Check sheet for the modelled part. Datum: model origin and axes. Units: mm. Face numbers are marked on the shaded views. A direction names the side the tool comes from. Round coordinates to 2 decimals unless told otherwise and drop trailing zeros. Write each loop counter-clockwise with the first axis right and the second up, starting at its lowest first coordinate (ties: lowest second). Pieces come first, ordered by that corner, then holes. Notation, with made-up numbers: (20, 48) - (72, 48) arc R12 cw to (72, 64) - close; hole circle Ø7 at (7, 37.25). An arc over 180 degrees is marked (long way). Answer as a JSON object with one key per item and string values. Group by question number.
Item 1: Release check for a two-part mould opening along X. For the marked faces 3, 4 and 5 record: pulls with the +X half, pulls with the -X half, needs draft (parallel to the pull), parting line crosses it, or undercut.
Item 2: Sectioned sample at A-A on z = 38. Record the boundary of the cut face in (x, y).
Item 3: Sectioned sample at C-C on x = -7.5. Record the boundary of the cut face in (y, z) (3 decimals).
Item 4: Set-up check for the marked faces 1 and 2: record each of +Z, -Z, +X, -X, +Y, -Y from which the full face is reachable in a straight line by a thin tool's end or side.
Item 5: Sectioned sample at B-B on y = -16.5. Record the boundary of the cut face in (x, z) (3 decimals).
Item 6: Gauge pin test, flat ends, axial feed: P1, Ø1, axis at x = 20, z = 42.5, coming from the +Y side; P2, Ø1, axis at x = -14, y = -16.5, coming from the +Z side (3 decimals). Record the tip position at first contact, or that the pin passes through.
Item 7: Thickness scan on line 1 (X direction, y = -4.5, z = 68); line 2 (Y direction, x = 42.5, z = 33); line 3 (Z direction, x = -27, y = -39) (3 decimals). Record the ranges inside material, lowest first.
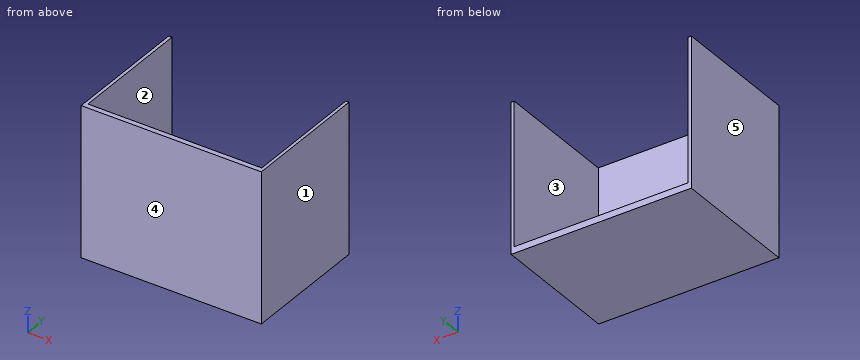
```python
from build123d import *

# Parameters (mm, degrees)
SKETCH1_W           = 88.9
SKETCH1_H           = 63.5
BOSS_EXTRUDE1_DEPTH = 3.175
SKETCH4_W           = 1.617754759
SKETCH4_H           = 63.5
BOSS_EXTRUDE2_DEPTH = 70.612
SKETCH5_W           = 1.524
SKETCH5_H           = 63.5
BOSS_EXTRUDE3_DEPTH = 70.612
SKETCH6_W           = 88.9
SKETCH6_H           = 73.787
BOSS_EXTRUDE4_DEPTH = 2.54


with BuildPart() as part:
    # Sketch1 → Boss-Extrude1 (new body)
    with BuildSketch(Plane.XY):
        with Locations((11.755371901, -15.035330579)):
            Rectangle(SKETCH1_W, SKETCH1_H)
    extrude(amount=BOSS_EXTRUDE1_DEPTH)

    # Sketch4 → Boss-Extrude2 (add)
    with BuildSketch(Plane.XY.offset(3.175)):
        with Locations((-31.88575072, -15.035330579)):
            Rectangle(SKETCH4_W, SKETCH4_H)
    extrude(amount=BOSS_EXTRUDE2_DEPTH)

    # Sketch5 → Boss-Extrude3 (add)
    with BuildSketch(Plane.XY.offset(3.175)):
        with Locations((55.443371901, -15.035330579)):
            Rectangle(SKETCH5_W, SKETCH5_H)
    extrude(amount=BOSS_EXTRUDE3_DEPTH)

    # Sketch6 → Boss-Extrude4 (add)
    with BuildSketch(Plane.XZ.offset(46.785330579)):
        with Locations((11.755371901, 36.8935)):
            Rectangle(SKETCH6_W, SKETCH6_H)
    extrude(amount=-BOSS_EXTRUDE4_DEPTH)


solid = part.part
```
Completed:
{
 "1": {"face 3": "undercut", "face 4": "needs draft", "face 5": "pulls with the -X half"},
 "2": {"outline": "(-32.69, -46.79) - (56.21, -46.79) - (56.21, 16.71) - (54.68, 16.71) - (54.68, -44.25) - (-31.08, -44.25) - (-31.08, 16.71) - (-32.69, 16.71) - close"},
 "3": {"outline": "(-46.785, 0) - (16.715, 0) - (16.715, 3.175) - (-44.245, 3.175) - (-44.245, 73.787) - (-46.785, 73.787) - close"},
 "4": {"face 1": "+Z, -Z, +X, +Y, -Y", "face 2": "+Z, +Y"},
 "5": {"outline": "(-32.695, 0) - (56.205, 0) - (56.205, 73.787) - (54.681, 73.787) - (54.681, 3.175) - (-31.077, 3.175) - (-31.077, 73.787) - (-32.695, 73.787) - close"},
 "6": {"P1": "y = -44.25", "P2": "z = 3.175"},
 "7": {"line 1": "-32.69 to -31.08, 54.68 to 56.21", "line 2": "-46.79 to -44.25", "line 3": "0 to 3.175"}
}
